```python
from build123d import *

# Parameters (mm, degrees)
SKETCH_1_R      = 46
SKETCH_1_R_2    = 1.55
SKETCH_1_R_3    = 34.05
EXTRUDE_1_DEPTH = 5


with BuildPart() as part:
    # 草图1 → 凸台-拉伸1 (new body)
    with BuildSketch(Plane.XY.offset(2.5)):
        Circle(SKETCH_1_R)
        with Locations((33.341978046, 19.25)):
            Circle(SKETCH_1_R_2, mode=Mode.SUBTRACT)
        with Locations((33.341978046, -19.25)):
            Circle(SKETCH_1_R_2, mode=Mode.SUBTRACT)
        with Locations((0, -38.5)):
            Circle(SKETCH_1_R_2, mode=Mode.SUBTRACT)
        with Locations((-33.341978046, -19.25)):
            Circle(SKETCH_1_R_2, mode=Mode.SUBTRACT)
        with Locations((-33.341978046, 19.25)):
            Circle(SKETCH_1_R_2, mode=Mode.SUBTRACT)
        with Locations((0, 38.5)):
            Circle(SKETCH_1_R_2, mode=Mode.SUBTRACT)
        Circle(SKETCH_1_R_3, mode=Mode.SUBTRACT)
        with BuildLine():
            ThreePointArc((-5.298278059, 36.618687164), (-18.5, 32.04293994), (-29.063574308, 22.897786978))
            ThreePointArc((-29.063574308, 22.897786978), (-31.170115981, 22.647822626), (-31.420080332, 24.7543643))
            ThreePointArc((-31.420080332, 24.7543643), (-20, 34.641016151), (-5.727868172, 39.587769907))
            ThreePointArc((-5.727868172, 39.587769907), (-4.028531744, 38.318023592), (-5.298278059, 36.618687164))
        make_face(mode=Mode.SUBTRACT)
        with BuildLine():
            ThreePointArc((29.063574308, 22.897786978), (18.5, 32.04293994), (5.298278059, 36.618687164))
            ThreePointArc((5.298278059, 36.618687164), (4.028531744, 38.318023592), (5.727868172, 39.587769907))
            ThreePointArc((5.727868172, 39.587769907), (20, 34.641016151), (31.420080332, 24.7543643))
            ThreePointArc((31.420080332, 24.7543643), (31.170115981, 22.647822626), (29.063574308, 22.897786978))
        make_face(mode=Mode.SUBTRACT)
        with BuildLine():
            ThreePointArc((34.361852367, -13.720900186), (37, 0), (34.361852367, 13.720900186))
            ThreePointArc((34.361852367, 13.720900186), (35.198647725, 15.670200965), (37.147948505, 14.833405607))
            ThreePointArc((37.147948505, 14.833405607), (40, 0), (37.147948505, -14.833405607))
            ThreePointArc((37.147948505, -14.833405607), (35.198647725, -15.670200965), (34.361852367, -13.720900186))
        make_face(mode=Mode.SUBTRACT)
        with BuildLine():
            ThreePointArc((5.298278059, -36.618687164), (18.5, -32.04293994), (29.063574308, -22.897786978))
            ThreePointArc((29.063574308, -22.897786978), (31.170115981, -22.647822626), (31.420080332, -24.7543643))
            ThreePointArc((31.420080332, -24.7543643), (20, -34.641016151), (5.727868172, -39.587769907))
            ThreePointArc((5.727868172, -39.587769907), (4.028531744, -38.318023592), (5.298278059, -36.618687164))
        make_face(mode=Mode.SUBTRACT)
        with BuildLine():
            ThreePointArc((-29.063574308, -22.897786978), (-18.5, -32.04293994), (-5.298278059, -36.618687164))
            ThreePointArc((-5.298278059, -36.618687164), (-4.028531744, -38.318023592), (-5.727868172, -39.587769907))
            ThreePointArc((-5.727868172, -39.587769907), (-20, -34.641016151), (-31.420080332, -24.7543643))
            ThreePointArc((-31.420080332, -24.7543643), (-31.170115981, -22.647822626), (-29.063574308, -22.897786978))
        make_face(mode=Mode.SUBTRACT)
        with BuildLine():
            ThreePointArc((-34.361852367, 13.720900186), (-37, 0), (-34.361852367, -13.720900186))
            ThreePointArc((-34.361852367, -13.720900186), (-35.198647725, -15.670200965), (-37.147948505, -14.833405607))
            ThreePointArc((-37.147948505, -14.833405607), (-40, 0), (-37.147948505, 14.833405607))
            ThreePointArc((-37.147948505, 14.833405607), (-35.198647725, 15.670200965), (-34.361852367, 13.720900186))
        make_face(mode=Mode.SUBTRACT)
    extrude(amount=-EXTRUDE_1_DEPTH)


solid = part.part
```
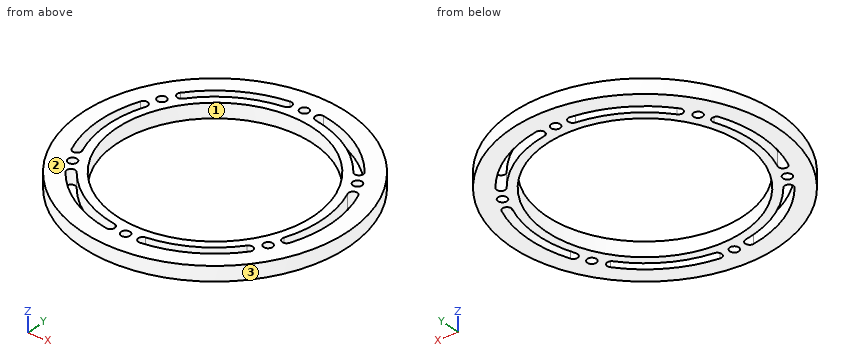
Model file for the job. Use its own axes, mm. Face numbers are marked on the shaded views. Coordinates: 2 decimals unless noted, no trailing zeros. Order: outer loops, then holes, each group sorted by start corner. A loop starts at its lowest first (then second) coordinate and runs counter-clockwise, first axis right, second up. Notation, with made-up numbers: (-3.75, 21) - (52.25, 21) arc R13 cw to (52.25, 35) - close; hole circle Ø3 at (0.25, -28.5). An arc over 180 degrees is marked (long way). Return JSON: item names as keys, results as strings. Group by question number.
1) Saw through at C-C, the plane x = 8. Write the cut outline in (y, z), plus the area to 3 significant figures.
2) Saw through at B-B, the plane z = 1.45. Count the separate pieces of the cut face and the enclosed holes in it, plus the area to 3 significant figures.
3) Flat gauge pins, fed straight in: P1, Ø3, axis at x = -6.5, z = -1.5, coming from the -Y side; P2, Ø2.5, axis at x = 0, y = 38.5, coming from the +Z side; P3, Ø3, axis at x = 15.5, z = -0.5, coming from the +Y side. Where does each tip first touch, or does it go through?
4) Mould opens along Y. For the marked faces 1, 2 and 3 say: released by +Y, released by -Y, zero draft, split by the parting line, or undercut.
5) Probe line 1 (X direction, y = 9, z = 0.9); line 2 (Y direction, x = -24, z = 1.65); line 3 (Y direction, x = 26.5, z = 2.35). List the from-to ranges inside material, lowest first. Write a range as from..to.
6) Saw through at A-A, the plane y = 0. Write the cut outline in (x, z), plus the area to 3 significant figures.
Values found:
{
 "1": {"outline": "(-45.3, -2.5) - (-39.19, -2.5) - (-39.19, 2.5) - (-45.3, 2.5) - close; (-36.12, -2.5) - (-33.1, -2.5) - (-33.1, 2.5) - (-36.12, 2.5) - close; (33.1, -2.5) - (36.12, -2.5) - (36.12, 2.5) - (33.1, 2.5) - close; (39.19, -2.5) - (45.3, -2.5) - (45.3, 2.5) - (39.19, 2.5) - close", "area": "91.4 mm²"},
 "2": {"separate pieces": "1", "enclosed holes": "13", "area": "2,390 mm²"},
 "3": {"P1": "stops at y = -45.73", "P2": "passes through", "P3": "stops at y = 43.82"},
 "4": {"face 1": "undercut", "face 2": "zero draft", "face 3": "split by the parting line"},
 "5": {"line 1": "x = -45.11..-38.97, -35.89..-32.84, 32.84..35.89, 38.97..45.11", "line 2": "y = -39.24..-32, -28.16..-24.15, 24.15..28.16, 32..39.24", "line 3": "y = -37.6..-29.96, -25.82..-21.38, 21.38..25.82, 29.96..37.6"},
 "6": {"outline": "(-46, -2.5) - (-40, -2.5) - (-40, 2.5) - (-46, 2.5) - close; (-37, -2.5) - (-34.05, -2.5) - (-34.05, 2.5) - (-37, 2.5) - close; (34.05, -2.5) - (37, -2.5) - (37, 2.5) - (34.05, 2.5) - close; (40, -2.5) - (46, -2.5) - (46, 2.5) - (40, 2.5) - close", "area": "89.5 mm²"}
}
